from build123d import *

# Parameters (mm, degrees)
SKETCH_R        = 23.15
PAD_DEPTH       = 5
SKETCH001_R     = 25
PAD001_DEPTH    = 3
CHAMFER_SIZE    = 2
SKETCH002_R     = 22
POCKET_DEPTH    = 6
CHAMFER001_SIZE = 2


with BuildPart() as part:
    # Sketch → Pad (new body)
    with BuildSketch(Plane.XY):
        Circle(SKETCH_R)
    extrude(amount=PAD_DEPTH)

    # Sketch001 (on Face3 of Pad) → Pad001 (join)
    with BuildSketch(Plane.XY.offset(5)):
        Circle(SKETCH001_R)
    extrude(amount=PAD001_DEPTH)

    # Chamfer
    chamfer_edges = [part.edges().sort_by_distance(p)[0] for p in [
        (-25, 0, 8),
    ]]
    chamfer(chamfer_edges, length=CHAMFER_SIZE)

    # Sketch002 (on Face6 of Chamfer) → Pocket (cut)
    with BuildSketch(Plane(origin=(0, 0, 0), x_dir=(1, 0, 0), z_dir=(0, 0, -1))):
        Circle(SKETCH002_R)
    extrude(amount=-POCKET_DEPTH, mode=Mode.SUBTRACT)

    # Chamfer001
    chamfer001_edges = [part.edges().sort_by_distance(p)[0] for p in [
        (-22, 0, 6),
    ]]
    chamfer(chamfer001_edges, length=CHAMFER001_SIZE)


with BuildPart() as part_1:
    # Body placement: moved
    add(part.part.moved(Location((0, 0, -15))))


solid = part_1.part
CAD build for the part. Positions are in the model's coordinates, mm. A direction names the side the tool comes from. Round coordinates to 2 decimals unless told otherwise and drop trailing zeros. Write each loop counter-clockwise with the first axis right and the second up, starting at its lowest first coordinate (ties: lowest second). Pieces come first, ordered by that corner, then holes. Notation, with made-up numbers: M 15,51 L 36,51 A11 ccw 36,71 Z; hole C 75.25,74.5 d8. An arc over 180 degrees is marked long. Use a Markdown table: item, result. Add a question column.
1. Flat gauge pins, fed straight in: P1, Ø1.5, axis at y = -9, z = -8.5, coming from the -X side; P2, Ø2, axis at x = 14.5, y = -2, coming from the -Z side; P3, Ø1.5, axis at x = 7, z = -9, coming from the +Y side. Where does each tip first touch, or does it go through?
2. Slice it at C-C on z = -13. Give the cut face in (x, y), then the cut area to 3 significant figures.
3. 3-axis set-ups, long thin cutter, end or side, ignore diameter. For faces 4 (the face through (-4.769, 21.477, -13.028)), 5 (the face through (23.846, 7.509, -9.507)): which of +Z, -Z, +X, -X, +Y, -Y reach the whole face in a straight line?
4. Drill centre lines: probe 1 along Y at (x, z) = (0, -13.9); probe 2 along Z at (x, y) = (8.5, 14.5); probe 3 along Y at (x, z) = (-10, -9.25). Where is each one in solid material? Low to high.
5. Slice it at D-D on z = -8. Give the cut face in (x, y).
6. Slice it at A-A on x = 0. Give the cut face in (y, z).
7. Pull direction Y, two halves, no side cores. Call faces 1 (the face through (0, 0, -9)), 2 (the face through (0, 0, -7)), 3 (the face through (-23.128, 1.018, -12.535)): released by +Y, released by -Y, zero draft, split by the parting line, or undercut.
Reply:
| question | item | result |
|---|---|---|
| 1 | P1 | stops at x = -23.53 |
| 1 | P2 | stops at z = -9 |
| 1 | P3 | stops at y = 24.21 |
| 2 | outline | C 0,0 d46.3; hole C 0,0 d44 |
| 2 | area | 163 mm^2 |
| 3 | face 4 | -Z |
| 3 | face 5 | +Z, -Z |
| 4 | probe 1 | y = -23.15 to -22, 22 to 23.15 |
| 4 | probe 2 | z = -9 to -7 |
| 4 | probe 3 | y = -22.91 to -17.61, 17.61 to 22.91 |
| 5 | outline | C 0,0 d48 |
| 6 | outline | M -25,-10 L -23.15,-10 L -23.15,-15 L -22,-15 L -22,-11 L -20,-9 L 20,-9 L 22,-11 L 22,-15 L 23.15,-15 L 23.15,-10 L 25,-10 L 25,-9 L 23,-7 L -23,-7 L -25,-9 Z |
| 7 | face 1 | undercut |
| 7 | face 2 | zero draft |
| 7 | face 3 | split by the parting line |
